```python
from build123d import *

# Parameters (mm, degrees)
SKIZZE1_R                       = 5.1
SKIZZE1_R_2                     = 0.5
AUFSATZ_LINEAR_AUSTRAGEN1_DEPTH = 1.9
SKIZZE2_W                       = 4
SKIZZE2_H                       = 4
AUFSATZ_LINEAR_AUSTRAGEN2_DEPTH = 1.1
VERRUNDUNG1_R                   = 0.3


with BuildPart() as part:
    # Skizze1 → Aufsatz-Linear austragen1 (new body)
    with BuildSketch(Plane(origin=(0, 0, 0), x_dir=(1, 0, 0), z_dir=(0, 1, 0))):
        with Locations(Location((0, 0, 0), (0, 0, 90))):
            Circle(SKIZZE1_R)
        with Locations(Location((0, 4.2, 0), (0, 0, 270))):
            Circle(SKIZZE1_R_2, mode=Mode.SUBTRACT)
        with Locations(Location((2.194493972, 3.58108869, 0), (0, 0, 270))):
            Circle(SKIZZE1_R_2, mode=Mode.SUBTRACT)
        with Locations(Location((3.742227402, 1.906760099, 0), (0, 0, 270))):
            Circle(SKIZZE1_R_2, mode=Mode.SUBTRACT)
        with Locations(Location((-3.742227402, 1.906760099, 0), (0, 0, 90))):
            Circle(SKIZZE1_R_2, mode=Mode.SUBTRACT)
        with Locations(Location((-2.194493972, 3.58108869, 0), (0, 0, 90))):
            Circle(SKIZZE1_R_2, mode=Mode.SUBTRACT)
    extrude(amount=AUFSATZ_LINEAR_AUSTRAGEN1_DEPTH)

    # Skizze2 → Aufsatz-Linear austragen2 (add)
    with BuildSketch(Plane(origin=(0, 1.9, 0), x_dir=(1, 0, 0), z_dir=(0, 1, 0))):
        Rectangle(SKIZZE2_W, SKIZZE2_H)
    extrude(amount=AUFSATZ_LINEAR_AUSTRAGEN2_DEPTH)

    # Verrundung1
    verrundung1_edges = [part.edges().sort_by_distance(p)[0] for p in [
        (2, 2.45, 2),
        (2, 2.45, -2),
        (-2, 2.45, -2),
        (-2, 2.45, 2),
    ]]
    fillet(verrundung1_edges, radius=VERRUNDUNG1_R)


solid = part.part
```
Can you work these out from the model? Positions are in its coordinate system, mm. A direction names the side the tool comes from. Round coordinates to 2 decimals unless told otherwise and drop trailing zeros. Order: outer loops, then holes, each group sorted by start corner. A loop starts at its lowest first (then second) coordinate and runs counter-clockwise, first axis right, second up. Notation, with made-up numbers: (-8.75, -34) -> (26.25, -34) arc R13 cw to (26.25, -27) -> close; hole circle Ø2 at (31, 3.25). An arc over 180 degrees is marked (long way). Return JSON: item names as keys, results as strings. Group by question number.
1. If we section it at A-A, the plane x = 0: Write out the boundary of the cut face in (y, z).
2. If we section it at B-B, the plane z = 0: Write out the boundary of the cut face in (x, y), then the cut area to 3 significant figures.
3. Will these pins go through, and if not, where does the flat tip stop? pin 1 (4 mm diameter, centred on x = -3, z = 3.5, fed in from -Y); pin 2 (0.9 mm diameter, centred on x = 0, y = 2.5, fed in from -Z); pin 3 (0.9 mm diameter, centred on y = 2.5, z = -1, fed in from +X); pin 4 (1 mm diameter, centred on y = 1.5, z = -3, fed in from -X).
4. We'd pull the mould along Y, two halves only. Please class faces 5 (the face through (2.2, 1.9, 0.1)), 6 (the face through (0, 0, 0)), 7 (the face through (1.706, 0.937, -3.689)): released by +Y, released by -Y, zero draft, split by the parting line, or undercut.
5. Which directions (+Z, -Z, +X, -X, +Y, -Y) give clear straight access to the entire face, cutting with the end or side of a thin tool? Please do faces 1 (the face through (0, 2.4, 2)), 2 (the face through (-2, 2.4, 0)), 3 (the face through (2, 2.4, 0)), 4 (the face through (0, 2.4, -2)).
6. If we section it at C-C, the plane y = 2.15: Write out the boundary of the cut face in (x, z), then the cut area to 3 significant figures.
7. I need wall thicknesses on line 1 (X direction, y = 2.05, z = -1.5); line 2 (X direction, y = 1.2, z = -2); line 3 (Y direction, x = -0.75, z = 2.5). Which ranges of each line are inside material? Lowest first, please. Write a range as [from, to].
8. If we section it at D-D, the plane z = -4.2: Write out the boundary of the cut face in (x, y), then the cut area to 3 significant figures.
Output values:
{
 "1": {"outline": "(0, -5.1) -> (1.9, -5.1) -> (1.9, -4.7) -> (0, -4.7) -> close; (0, -3.7) -> (1.9, -3.7) -> (1.9, -2) -> (3, -2) -> (3, 2) -> (1.9, 2) -> (1.9, 5.1) -> (0, 5.1) -> close"},
 "2": {"outline": "(-5.1, 0) -> (5.1, 0) -> (5.1, 1.9) -> (2, 1.9) -> (2, 3) -> (-2, 3) -> (-2, 1.9) -> (-5.1, 1.9) -> close", "area": "23.8 mm²"},
 "3": {"pin 1": "y = 0", "pin 2": "z = -2", "pin 3": "x = 2", "pin 4": "x = -4.45"},
 "4": {"face 5": "released by +Y", "face 6": "released by -Y", "face 7": "zero draft"},
 "5": {"face 1": "+Z, +X, -X, +Y", "face 2": "+Z, -Z, -X, +Y", "face 3": "+Z, -Z, +X, +Y", "face 4": "-Z, +X, -X, +Y"},
 "6": {"outline": "(-2, -1.7) arc R0.3 ccw to (-1.7, -2) -> (1.7, -2) arc R0.3 ccw to (2, -1.7) -> (2, 1.7) arc R0.3 ccw to (1.7, 2) -> (-1.7, 2) arc R0.3 ccw to (-2, 1.7) -> close", "area": "15.9 mm²"},
 "7": {"line 1": "[-2, 2]", "line 2": "[-4.69, -4.23], [-3.25, 3.25], [4.23, 4.69]", "line 3": "[0, 1.9]"},
 "8": {"outline": "(-2.89, 0) -> (-0.5, 0) -> (-0.5, 1.9) -> (-2.89, 1.9) -> close; (0.5, 0) -> (2.89, 0) -> (2.89, 1.9) -> (0.5, 1.9) -> close", "area": "9.09 mm²"}
}
